Design review of the part built by this model. Coordinates are the model's own, in mm. Coordinates: 2 decimals unless noted, no trailing zeros. Loops run counter-clockwise (first coordinate to the right, second up) from the corner with the lowest first, then second, coordinate; pieces in that order, holes last. Notation, with made-up numbers: M 83.25,-37.75 L 110.25,-37.75 A7 ccw 110.25,-31.75 Z; hole C 54,57 d3. An arc over 180 degrees is marked long. One line per item, written item: value.
```python
from build123d import *

# Parameters (mm, degrees)
F1_DEPTH = 25.4
F3_DEPTH = 12.7


with BuildPart() as f1:
    # F0 (on Front) → F1 (new body)
    with BuildSketch(Plane.XZ):
        with BuildLine():
            Line((1.674858, 12.589077), (0, 12.7))
            ThreePointArc((0, 12.7), (-12.7, 0), (0, -12.7))
            Line((0, -12.7), (1.674858, -12.589077))
            ThreePointArc((1.674858, -12.589077), (9.554075, -8.367177), (12.7, 0))
            ThreePointArc((12.7, 0), (9.554075, 8.367177), (1.674858, 12.589077))
        make_face()
        with BuildLine():
            ThreePointArc((1.674858, 12.589077), (0.839264, 12.672239), (0, 12.7))
            Line((0, 12.7), (1.674858, 12.589077))
        make_face()
        with BuildLine():
            Line((1.674858, -12.589077), (0, -12.7))
            ThreePointArc((0, -12.7), (0.839264, -12.672239), (1.674858, -12.589077))
        make_face()
        with BuildLine():
            Line((48.254448, 9.504179), (1.674858, 12.589077))
            ThreePointArc((1.674858, 12.589077), (9.554075, 8.367177), (12.7, 0))
            ThreePointArc((12.7, 0), (9.554075, -8.367177), (1.674858, -12.589077))
            Line((1.674858, -12.589077), (48.254448, -9.504179))
            ThreePointArc((48.254448, -9.504179), (38.1, 0), (48.254448, 9.504179))
        make_face()
        with BuildLine():
            ThreePointArc((57.15, 0), (54.579176, 6.508845), (48.254448, 9.504179))
            ThreePointArc((48.254448, 9.504179), (38.1, 0), (48.254448, -9.504179))
            ThreePointArc((48.254448, -9.504179), (54.579176, -6.508845), (57.15, 0))
        make_face()
    extrude(amount=-F1_DEPTH)

    # F2 (on Top) → F3 (cut, symmetric)
    with BuildSketch(Plane.XY):
        Polygon((25.4, 0), (57.15, 0), (57.15, 11.556055), align=None)
    extrude(amount=F3_DEPTH, both=True, mode=Mode.SUBTRACT)


solid = f1.part
```
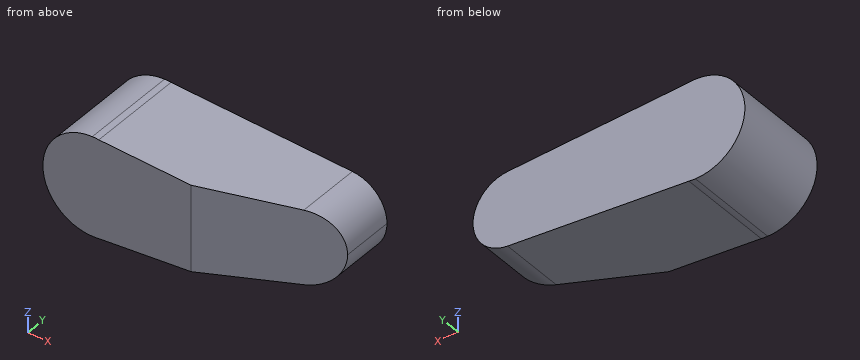
(1) We need section B-B on z = -1.5. State the section outline as (x, y) points, then the cut area to 3 significant figures.
Reply:
outline: M -12.61,0 L 25.4,0 L 57.03,11.51 L 57.03,25.4 L -12.61,25.4 Z
area: 1,590 mm2
(2) To check wall thickness, follow line 1 along X through (y, z) = (20, -5); line 2 along Z through (x, y) = (37.5, 7); line 3 along Z through (x, y) = (49, 16.25). State the ranges of each line that lie inside material, in increasing order. Write a range as [from, to].
Reply:
line 1: x = [-11.67, 55.73]
line 2: z = [-10.22, 10.22]
line 3: z = [-9.43, 9.43]
(3) Insertion check: pin 1 (3 mm diameter, centred on x = 33.5, y = 21.5, fed in from +Z); pin 2 (6 mm diameter, centred on x = 20.5, y = 13.5, fed in from -Z); pin 3 (4 mm diameter, centred on y = 18, z = 3.5, fed in from +X). Each pin has a flat end and moves straight along its axis. Give the tip position at first contact, or say it passes through.
Reply:
pin 1: stops at z = 10.58
pin 2: stops at z = -11.54
pin 3: stops at x = 57.03
(4) We need section D-D on z = 6.75. State the section outline as (x, y) points.
Reply:
outline: M -10.76,0 L 25.4,0 L 54.35,10.54 L 54.35,25.4 L -10.76,25.4 Z
(5) We need section C-C on x = 17. State the section outline as (y, z) points, then the cut area to 3 significant figures.
Reply:
outline: M 0,-11.57 L 25.4,-11.57 L 25.4,11.57 L 0,11.57 Z
area: 588 mm2
(6) We need section A-A on y = 12.75. State the section outline as (x, z) points (3 decimals), then the cut area to 3 significant figures.
Reply:
outline: M 0,-12.7 A12.7 ccw 1.675,-12.589 L 48.254,-9.504 A9.525 ccw 48.254,9.504 L 1.675,12.589 A12.7 ccw 0,12.7 A12.7 ccw Z
area: 1,460 mm2
